Source: CAD feature listing. Evaluate the final solid. Frame: model axes, mm. A direction names the side the tool comes from. Round coordinates to 2 decimals unless told otherwise and drop trailing zeros. Loops run counter-clockwise (first coordinate to the right, second up) from the corner with the lowest first, then second, coordinate; pieces in that order, holes last. Notation, with made-up numbers: M 27,41 L 33,41 A23 cw 33,70 Z; hole C 85.25,1.25 d3. An arc over 180 degrees is marked long. Answer as a JSON object with one key per item and string values.
from build123d import *

# Parameters (mm, degrees)
SKETCH1_W                                       = 53.34
SKETCH1_H                                       = 66.04
SKETCH1_R                                       = 2.5527
SKETCH1_R_2                                     = 2.60985
SKETCH1_R_3                                     = 2.7051
SKETCH1_R_4                                     = 2.4003
SKETCH1_R_5                                     = 2.3114
SKETCH1_R_6                                     = 2.2479
SKETCH1_R_7                                     = 1.89865
SKETCH1_R_8                                     = 1.9558
SKETCH1_R_9                                     = 2.0193
SKETCH1_R_10                                    = 1.9
SKETCH1_R_11                                    = 1.8
SKETCH1_R_12                                    = 1.7
SKETCH1_R_13                                    = 1.1
SKETCH1_R_14                                    = 1.2
SKETCH1_R_15                                    = 1.3
SKETCH1_R_16                                    = 2.4892
SKETCH1_R_17                                    = 2.15265
SKETCH1_R_18                                    = 1.8288
SKETCH1_R_19                                    = 1.6
BOSS_EXTRUDE1_DEPTH                             = 7.9375
LPATTERN1_COUNT                                 = 2
LPATTERN1_PITCH                                 = 50.8
CBORE_FOR_10_SOCKET_HEAD_CAP_SCREW1_D           = 4.9784
CBORE_FOR_10_SOCKET_HEAD_CAP_SCREW1_CBORE_D     = 9.525
CBORE_FOR_10_SOCKET_HEAD_CAP_SCREW1_CBORE_DEPTH = 4.826
CBORE_FOR_8_SOCKET_HEAD_CAP_SCREW1_D            = 4.3053
CBORE_FOR_8_SOCKET_HEAD_CAP_SCREW1_CBORE_D      = 7.9375
CBORE_FOR_8_SOCKET_HEAD_CAP_SCREW1_CBORE_DEPTH  = 4.1656
CBORE_FOR_6_SOCKET_HEAD_CAP_SCREW1_D            = 3.6576
CBORE_FOR_6_SOCKET_HEAD_CAP_SCREW1_CBORE_D      = 7.14502
CBORE_FOR_6_SOCKET_HEAD_CAP_SCREW1_CBORE_DEPTH  = 3.5052
CBORE_FOR_M3_SHCS1_D                            = 3.2
CBORE_FOR_M3_SHCS1_CBORE_D                      = 6.5
CBORE_FOR_M3_SHCS1_CBORE_DEPTH                  = 3
CBORE_FOR_M2_SHCS1_D                            = 2.2
CBORE_FOR_M2_SHCS1_CBORE_D                      = 4.4
CBORE_FOR_M2_SHCS1_CBORE_DEPTH                  = 2
FILLET1_R                                       = 7.62


with BuildPart() as part:
    # Sketch1 → Boss-Extrude1 (new body)
    with BuildSketch(Plane(origin=(0, 0, 0), x_dir=(1, 0, 0), z_dir=(0, 1, 0))):
        with Locations((26.67, 33.02)):
            Rectangle(SKETCH1_W, SKETCH1_H)
        with Locations(Location((20.32, 58.42, 0), (0, 0, 270))):
            Circle(SKETCH1_R, mode=Mode.SUBTRACT)
        with Locations(Location((33.02, 58.42, 0), (0, 0, 270))):
            Circle(SKETCH1_R_2, mode=Mode.SUBTRACT)
        with Locations(Location((45.72, 58.42, 0), (0, 0, 270))):
            Circle(SKETCH1_R_3, mode=Mode.SUBTRACT)
        with Locations(Location((45.72, 45.72, 0), (0, 0, 270))):
            Circle(SKETCH1_R_4, mode=Mode.SUBTRACT)
        with Locations(Location((33.02, 45.72, 0), (0, 0, 270))):
            Circle(SKETCH1_R_5, mode=Mode.SUBTRACT)
        with Locations(Location((20.32, 45.72, 0), (0, 0, 270))):
            Circle(SKETCH1_R_6, mode=Mode.SUBTRACT)
        with Locations(Location((20.32, 33.02, 0), (0, 0, 270))):
            Circle(SKETCH1_R_7, mode=Mode.SUBTRACT)
        with Locations(Location((33.02, 33.02, 0), (0, 0, 270))):
            Circle(SKETCH1_R_8, mode=Mode.SUBTRACT)
        with Locations(Location((45.72, 33.02, 0), (0, 0, 270))):
            Circle(SKETCH1_R_9, mode=Mode.SUBTRACT)
        with Locations(Location((45.72, 20.32, 0), (0, 0, 270))):
            Circle(SKETCH1_R_10, mode=Mode.SUBTRACT)
        with Locations(Location((33.02, 20.32, 0), (0, 0, 270))):
            Circle(SKETCH1_R_11, mode=Mode.SUBTRACT)
        with Locations(Location((20.32, 20.32, 0), (0, 0, 270))):
            Circle(SKETCH1_R_12, mode=Mode.SUBTRACT)
        with Locations(Location((20.32, 7.62, 0), (0, 0, 270))):
            Circle(SKETCH1_R_13, mode=Mode.SUBTRACT)
        with Locations(Location((33.02, 7.62, 0), (0, 0, 270))):
            Circle(SKETCH1_R_14, mode=Mode.SUBTRACT)
        with Locations(Location((45.72, 7.62, 0), (0, 0, 270))):
            Circle(SKETCH1_R_15, mode=Mode.SUBTRACT)
        with Locations(Location((7.62, 58.42, 0), (0, 0, 270))):
            Circle(SKETCH1_R_16, mode=Mode.SUBTRACT)
        with Locations(Location((7.62, 45.72, 0), (0, 0, 270))):
            Circle(SKETCH1_R_17, mode=Mode.SUBTRACT)
        with Locations(Location((7.62, 33.02, 0), (0, 0, 270))):
            Circle(SKETCH1_R_18, mode=Mode.SUBTRACT)
        with Locations(Location((7.62, 7.62, 0), (0, 0, 270))):
            Circle(SKETCH1_R_13, mode=Mode.SUBTRACT)
        with Locations(Location((7.62, 20.32, 0), (0, 0, 270))):
            Circle(SKETCH1_R_19, mode=Mode.SUBTRACT)
    extrude(amount=-BOSS_EXTRUDE1_DEPTH)


with BuildPart() as lpattern1_1:
    # LPattern1: pattern copy
    add(part.part.moved(Location(Vector(1, 0, 0) * (1 * LPATTERN1_PITCH))))

    # Combine1: union part
    add(part.part)

    # CBORE for _10 Socket Head Cap Screw1 (through all)
    with Locations(Plane(origin=(0, 0, 0), x_dir=(1, 0, 0), z_dir=(0, 1, 0))):
        with Locations((7.62, 58.42), (20.32, 58.42), (33.02, 58.42), (45.72, 58.42)):
            CounterBoreHole(CBORE_FOR_10_SOCKET_HEAD_CAP_SCREW1_D / 2, CBORE_FOR_10_SOCKET_HEAD_CAP_SCREW1_CBORE_D / 2, CBORE_FOR_10_SOCKET_HEAD_CAP_SCREW1_CBORE_DEPTH)

    # CBORE for _8 Socket Head Cap Screw1 (through all)
    with Locations(Plane(origin=(0, 0, 0), x_dir=(1, 0, 0), z_dir=(0, 1, 0))):
        with Locations((7.62, 45.72), (20.32, 45.72), (33.02, 45.72), (45.72, 45.72)):
            CounterBoreHole(CBORE_FOR_8_SOCKET_HEAD_CAP_SCREW1_D / 2, CBORE_FOR_8_SOCKET_HEAD_CAP_SCREW1_CBORE_D / 2, CBORE_FOR_8_SOCKET_HEAD_CAP_SCREW1_CBORE_DEPTH)

    # CBORE for _6 Socket Head Cap Screw1 (through all)
    with Locations(Plane(origin=(0, 0, 0), x_dir=(1, 0, 0), z_dir=(0, 1, 0))):
        with Locations((7.62, 33.02), (20.32, 33.02), (33.02, 33.02), (45.72, 33.02)):
            CounterBoreHole(CBORE_FOR_6_SOCKET_HEAD_CAP_SCREW1_D / 2, CBORE_FOR_6_SOCKET_HEAD_CAP_SCREW1_CBORE_D / 2, CBORE_FOR_6_SOCKET_HEAD_CAP_SCREW1_CBORE_DEPTH)

    # CBORE for M3 SHCS1 (through all)
    with Locations(Plane(origin=(0, 0, 0), x_dir=(1, 0, 0), z_dir=(0, 1, 0))):
        with Locations((7.62, 20.32), (20.32, 20.32), (33.02, 20.32), (45.72, 20.32)):
            CounterBoreHole(CBORE_FOR_M3_SHCS1_D / 2, CBORE_FOR_M3_SHCS1_CBORE_D / 2, CBORE_FOR_M3_SHCS1_CBORE_DEPTH)

    # CBORE for M2 SHCS1 (through all)
    with Locations(Plane(origin=(0, 0, 0), x_dir=(1, 0, 0), z_dir=(0, 1, 0))):
        with Locations((7.62, 7.62), (20.32, 7.62), (33.02, 7.62), (45.72, 7.62)):
            CounterBoreHole(CBORE_FOR_M2_SHCS1_D / 2, CBORE_FOR_M2_SHCS1_CBORE_D / 2, CBORE_FOR_M2_SHCS1_CBORE_DEPTH)

    # Fillet1
    fillet1_edges = [lpattern1_1.edges().sort_by_distance(p)[0] for p in [
        (0, -3.96875, -66.04),
        (0, -3.96875, 0),
        (104.14, -3.96875, -66.04),
        (104.14, -3.96875, 0),
    ]]
    fillet(fillet1_edges, radius=FILLET1_R)


solid = lpattern1_1.part
Item 1: Contact query for flat-ended pins moving along their axis: pin 1 Ø6.5 at (x, z) = (45.72, -33.02) entering from +Y; pin 2 Ø6 at (x, z) = (45.72, -58.42) entering from +Y. Output: stop coordinate, or through.
Answer sheet:
{"pin 1": "stops at y = -3.51", "pin 2": "stops at y = -4.83"}
Item 2: Line query: probe 1 along Z at (x, y) = (7.62, -2.1); probe 2 along Z at (x, y) = (33.02, -1.6); probe 3 along X at (y, z) = (-0.5, -55.5). Output: solid intervals per line, ascending. Write a range as from..to.
Answer sheet:
{"probe 1": "z = -66.04..-63.18, -53.66..-49.69, -41.75..-36.59, -29.45..-23.57, -17.07..-8.72, -6.52..0", "probe 2": "z = -66.04..-63.18, -53.66..-49.69, -41.75..-36.59, -29.45..-23.57, -17.07..-9.82, -5.42..0", "probe 3": "x = 0..3.86, 11.38..16.56, 24.08..29.26, 36.78..41.96, 49.48..104.14"}
Item 3: Section B-B on z = -20.32. Give the number of separate pieces and of enclosed holes in the cut face, then the cut area to 3 significant figures.
Answer sheet:
{"separate pieces": "9", "enclosed holes": "0", "area": "568 mm²"}
Item 4: Access query for faces 1 (the cylindrical face through (41.94, -2.38, -55.52)), 2 (the cylindrical face through (8.169, -5.69, -31.276)). Directions: +Z, -Z, +X, -X, +Y, -Y. A direction counts if a zero-diameter tool reaches every point of the face in a straight line with its end or side. Return the directions, or none.
Answer sheet:
{"face 1": "+Y", "face 2": "+Y, -Y"}
Item 5: Section A-A on x = 83.82. Return the cut outline in (y, z), then the cut area to 3 significant figures.
Answer sheet:
{"outline": "M -7.94,-66.04 L 0,-66.04 L 0,-61.03 L -7.94,-61.03 Z; M -7.94,-55.81 L 0,-55.81 L 0,-48.03 L -7.94,-48.03 Z; M -7.94,-43.41 L 0,-43.41 L 0,-34.98 L -7.94,-34.98 Z; M -7.94,-31.06 L 0,-31.06 L 0,-22.12 L -7.94,-22.12 Z; M -7.94,-18.52 L 0,-18.52 L 0,-8.82 L -7.94,-8.82 Z; M -7.94,-6.42 L 0,-6.42 L 0,0 L -7.94,0 Z", "area": "367 mm²"}
